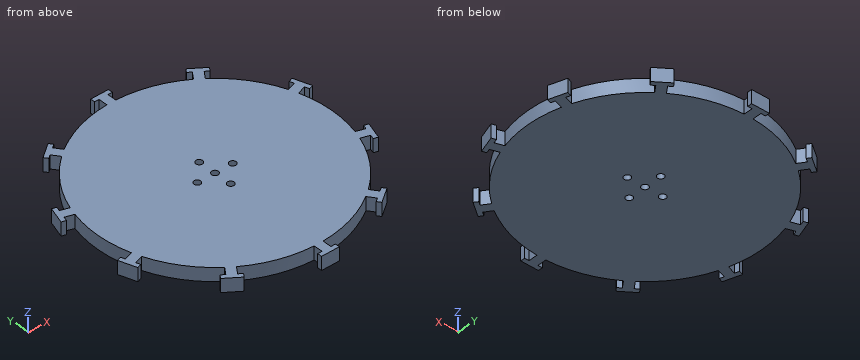
from build123d import *
from build123d.topology import SkipClean

# Parameters (mm, degrees)
SKETCH1_R           = 52.5
BOSS_EXTRUDE1_DEPTH = 2
BOSS_EXTRUDE2_DEPTH = 6
CIRPATTERN1_COUNT   = 10
SKETCH4_R           = 1.5
CUT_EXTRUDE2_DEPTH  = 10


with BuildPart() as part:
    # Sketch1 → Boss-Extrude1 (new body)
    with BuildSketch(Plane.XY):
        Circle(SKETCH1_R)
    extrude(amount=BOSS_EXTRUDE1_DEPTH)

    # Sketch6 → Boss-Extrude2 (add)
    with SkipClean():  # the faces are left unmerged after this step: merging them gives an invalid solid
        with BuildSketch(Plane.XY):
            with BuildLine():
                Line((-2, 52.46189093), (-2, 56.46189093))
                Line((-2, 56.46189093), (-4, 56.46189093))
                Line((-4, 56.46189093), (-4, 58.46189093))
                Line((-4, 58.46189093), (4, 58.46189093))
                Line((4, 58.46189093), (4, 56.46189093))
                Line((4, 56.46189093), (2, 56.46189093))
                Line((2, 56.46189093), (2, 52.46189093))
                ThreePointArc((2, 52.46189093), (0, -52.5), (-2, 52.46189093))
            make_face()
        boss_extrude2 = extrude(amount=BOSS_EXTRUDE2_DEPTH)

    # CirPattern1: Boss-Extrude2 ×10 about axis
    cirpattern1_axis = Axis((0, 0, 0), (0, 0, 1))
    for i in range(1, CIRPATTERN1_COUNT):
        add(boss_extrude2.rotate(cirpattern1_axis, i * 360 / CIRPATTERN1_COUNT))

    # Sketch4 → Cut-Extrude2 (cut, symmetric)
    with BuildSketch(Plane.XY.offset(6)):
        with Locations((0, 8)):
            Circle(SKETCH4_R)
        Circle(SKETCH4_R)
        with Locations((8, 0)):
            Circle(SKETCH4_R)
        with Locations((0, -8)):
            Circle(SKETCH4_R)
        with Locations((-8, 0)):
            Circle(SKETCH4_R)
    extrude(amount=CUT_EXTRUDE2_DEPTH, both=True, mode=Mode.SUBTRACT)


solid = part.part
Can you work these out from the model? Positions are in its coordinate system, mm. Give positions to 0.01 mm unless a question says otherwise; leave off trailing zeros. Loops run counter-clockwise (first coordinate to the right, second up) from the corner with the lowest first, then second, coordinate; pieces in that order, holes last. Notation, with made-up numbers: (8, 58) - (24, 58) arc R26 cw to (24, 85) - close; hole circle Ø2 at (-5.5, 43.25). An arc over 180 degrees is marked (long way). Return JSON: item names as keys, results as strings.
1. I want a section at B-B on y = 0. Please give me the cut outline in (x, z).
Output values:
{"outline": "(-52.5, 0) - (-9.5, 0) - (-9.5, 6) - (-52.5, 6) - close; (-6.5, 0) - (-1.5, 0) - (-1.5, 6) - (-6.5, 6) - close; (1.5, 0) - (6.5, 0) - (6.5, 6) - (1.5, 6) - close; (9.5, 0) - (52.5, 0) - (52.5, 6) - (9.5, 6) - close"}
2. If I drill on line 1 (Y direction, x = 0, z = 1.8); line 2 (Y direction, x = -30.5, z = 3); line 3 (X direction, y = 46.5, z = 0.55), over which ranges is the centre line in solid material (lowest first)?
Output values:
{"line 1": "y = -58.46 to -9.5, -6.5 to -1.5, 1.5 to 6.5, 9.5 to 58.46", "line 2": "y = -48.78 to -47.63, -45.38 to 45.38, 47.63 to 48.78", "line 3": "x = -35.46 to -31.31, -24.37 to 24.37, 31.31 to 35.46"}
3. I want a section at C-C on z = 2.5. Give the number of separate pieces and of enclosed holes in the cut face, and give its area (3 significant figures).
Output values:
{"separate pieces": "1", "enclosed holes": "5", "area": "8,940 mm²"}
4. I'm going to push flat-ended pins straight in: pin 1 Ø2 at (y, z) = (-58, 2) entering from +X; pin 2 Ø1.6 at (y, z) = (-57, 2.5) entering from -X; pin 3 Ø5 at (x, y) = (0, 0) entering from -Z; pin 4 Ø2.5 at (x, y) = (0, 8) entering from -Z. Where does each tip first touch, or does it pass through?
Output values:
{"pin 1": "stops at x = 4", "pin 2": "stops at x = -4", "pin 3": "stops at z = 0", "pin 4": "passes through"}
5. I want a section at A-A on x = 0. Please give me the cut outline in (y, z).
Output values:
{"outline": "(-58.46, 0) - (-9.5, 0) - (-9.5, 6) - (-58.46, 6) - close; (-6.5, 0) - (-1.5, 0) - (-1.5, 6) - (-6.5, 6) - close; (1.5, 0) - (6.5, 0) - (6.5, 6) - (1.5, 6) - close; (9.5, 0) - (58.46, 0) - (58.46, 6) - (9.5, 6) - close"}
6. I want a section at D-D on x = -12. Please give me the cut outline in (y, z), and give its area (3 significant figures).
Output values:
{"outline": "(-51.11, 0) - (51.11, 0) - (51.11, 6) - (-51.11, 6) - close", "area": "613 mm²"}
